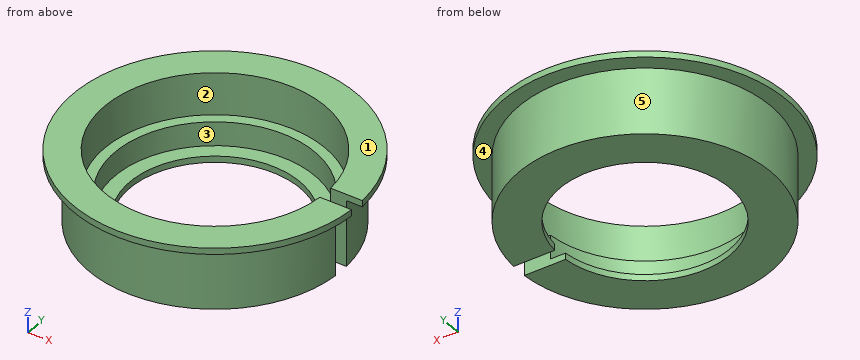
from build123d import *

# Parameters (mm, degrees)
F0_R      = 45
F1_DEPTH  = 23
F2_R      = 35
F3_DEPTH  = 13.4
F4_R      = 31.75
F5_DEPTH  = 7.6
F6_R      = 27
F7_DEPTH  = 2.001
F8_R      = 45
F8_R_2    = 40
F9_DEPTH  = 21
F10_W     = 30
F10_H     = 5
F11_DEPTH = 23.001


with BuildPart() as f1:
    # F0 (on Top) → F1 (new body)
    with BuildSketch(Plane.XY):
        Circle(F0_R)
    extrude(amount=F1_DEPTH)

    # F2 (on face) → F3 (cut)
    with BuildSketch(Plane.XY.offset(23)):
        Circle(F2_R)
    extrude(amount=-F3_DEPTH, mode=Mode.SUBTRACT)

    # F4 (on face) → F5 (cut)
    with BuildSketch(Plane.XY.offset(9.6)):
        Circle(F4_R)
    extrude(amount=-F5_DEPTH, mode=Mode.SUBTRACT)

    # F6 (on face) → F7 (cut, through all)
    with BuildSketch(Plane.XY.offset(2)):
        Circle(F6_R)
    extrude(amount=-F7_DEPTH, mode=Mode.SUBTRACT)

    # F8 (on face) → F9 (cut)
    with BuildSketch(Plane(origin=(0, 0, 0), x_dir=(1, 0, 0), z_dir=(0, 0, -1))):
        Circle(F8_R)
        Circle(F8_R_2, mode=Mode.SUBTRACT)
    extrude(amount=-F9_DEPTH, mode=Mode.SUBTRACT)

    # F10 (on face) → F11 (cut, through all)
    with BuildSketch(Plane.XY.offset(23)):
        with Locations((35, 0)):
            Rectangle(F10_W, F10_H)
    extrude(amount=-F11_DEPTH, mode=Mode.SUBTRACT)


solid = f1.part
Read the model definition and answer for the solid it produces. Units are mm, in the model's axes. Face numbers are marked on the shaded views. A direction names the side the tool comes from. Coordinates: 2 decimals unless noted, no trailing zeros. Loops run counter-clockwise (first coordinate to the right, second up) from the corner with the lowest first, then second, coordinate; pieces in that order, holes last.
Q1. The mould has two halves that part along Y. Classify the marked faces 3, 4 and 5: +Y half, -Y half, draft (parallel to the pull), parting line (faces both ways), or undercut.
Q2. The part is cut by section A-A on x = 0. Write down the section's boundary in (y, z).
Q3. Consider probe 1 along Y at (x, z) = (0, 14.75); probe 2 along Y at (x, z) = (0, 4.5); probe 3 along Z at (x, y) = (24, 19). Determine where each line is inside the solid, lowest interval first.
Q4. The part is cut by section B-B on y = 0. Write down the section's boundary in (x, z), and give its area (3 significant figures).
Q5. Each of these flat-tipped pins is pushed along its axis until it touches: pin 1 Ø5.5 at (x, z) = (39, 8) entering from +Y; pin 2 Ø2 at (x, z) = (-29.5, 14.5) entering from +Y; pin 3 Ø4 at (y, z) = (27.5, 7.5) entering from -X; pin 4 Ø8 at (x, y) = (-12, -15.5) entering from +Z. Where does it stop, or does it pass through?
Q6. Which of the six approach directions +Z, -Z, +X, -X, +Y, -Y give full straight-line access (tool end or side, diameter ignored) to the marked faces 1 and 2?
Q7. The part is cut by section C-C on y = -13. Write down the section's boundary in (x, z), and give its area (3 significant figures).
Q8. The part is cut by section D-D on z = 7.5. Write down the section's boundary in (x, y).
Results below:
1. face 3: undercut
1. face 4: draft
1. face 5: parting line
2. outline: (-45, 21) - (-40, 21) - (-40, 0) - (-27, 0) - (-27, 2) - (-31.75, 2) - (-31.75, 9.6) - (-35, 9.6) - (-35, 23) - (-45, 23) - close; (27, 0) - (40, 0) - (40, 21) - (45, 21) - (45, 23) - (35, 23) - (35, 9.6) - (31.75, 9.6) - (31.75, 2) - (27, 2) - close
3. probe 1: y = -40 to -35, 35 to 40
3. probe 2: y = -40 to -31.75, 31.75 to 40
3. probe 3: z = 0 to 2
4. outline: (-45, 21) - (-40, 21) - (-40, 0) - (-27, 0) - (-27, 2) - (-31.75, 2) - (-31.75, 9.6) - (-35, 9.6) - (-35, 23) - (-45, 23) - close
4. area: 166 mm2
5. pin 1: stops at y = 16.91
5. pin 2: stops at y = 28.07
5. pin 3: stops at x = -30.82
5. pin 4: passes through
6. face 1: +Z, +X, -X, +Y, -Y
6. face 2: +Z
7. outline: (-43.08, 21) - (-37.83, 21) - (-37.83, 0) - (-23.66, 0) - (-23.66, 2) - (-28.97, 2) - (-28.97, 9.6) - (-32.5, 9.6) - (-32.5, 23) - (-43.08, 23) - close; (23.66, 0) - (37.83, 0) - (37.83, 21) - (43.08, 21) - (43.08, 23) - (32.5, 23) - (32.5, 9.6) - (28.97, 9.6) - (28.97, 2) - (23.66, 2) - close
7. area: 355 mm2
8. outline: (31.65, -2.5) arc R31.75 cw (long way) to (31.65, 2.5) - (39.92, 2.5) arc R40 ccw (long way) to (39.92, -2.5) - close
